Design review of the part built by this model. Coordinates are the model's own, in mm. A direction names the side the tool comes from. Give positions to 0.01 mm unless a question says otherwise; leave off trailing zeros. Write each loop counter-clockwise with the first axis right and the second up, starting at its lowest first coordinate (ties: lowest second). Pieces come first, ordered by that corner, then holes. Notation, with made-up numbers: (34, 19) -> (58, 19) arc R9 ccw to (58, 34) -> close; hole circle Ø1 at (62, 3.5). An arc over 180 degrees is marked (long way). Use CSV: the item, a comma, the result in double quotes.
```python
from build123d import *

# Parameters (mm, degrees)
F0_W     = 34
F0_H     = 16
F1_DEPTH = 58
F3_DEPTH = 38.001
F4_W     = 34
F4_H     = 11
F5_DEPTH = 16
F7_DEPTH = 10
F8_R     = 8
F9_DEPTH = 22


with BuildPart() as f1:
    # F0 (on Top) → F1 (new body)
    with BuildSketch(Plane.XY):
        Polygon((0, 38), (0, 0), (34, 0), (75, 0), (75, 38), align=None)
        with Locations((17, -8)):
            Rectangle(F0_W, F0_H)
        Polygon((85.358984, 38), (75, 38), (75, 0), (120, 0), (120, 18), align=None)
    extrude(amount=F1_DEPTH)

    # F2 (on face) → F3 (cut, through all)
    with BuildSketch(Plane.XZ):
        Polygon((75, 58), (120, 32.019238), (120, 58), align=None)
    extrude(amount=-F3_DEPTH, mode=Mode.SUBTRACT)

    # F4 (on face) → F5 (cut, symmetric)
    with BuildSketch(Plane.XZ.offset(16)):
        with Locations((17, 52.5)):
            Rectangle(F4_W, F4_H)
    extrude(amount=F5_DEPTH, both=True, mode=Mode.SUBTRACT)

    # F6 (on face) → F7 (join, symmetric)
    with BuildSketch(Plane.XZ.offset(16)):
        Polygon((34, 47), (0, 47), (0, 0), (5, 0), (5, -6), (29, -6), (29, 0), (34, 0), align=None)
    extrude(amount=F7_DEPTH, both=True)

    # F8 (on face) → F9 (cut)
    with BuildSketch(Plane.XZ.offset(26)):
        with Locations((17, 23.5)):
            Circle(F8_R)
    extrude(amount=-F9_DEPTH, mode=Mode.SUBTRACT)


solid = f1.part
```
(1) For line 1 along X through (y, z) = (-20, 23); line 2 along Z through (x, y) = (17, -9.5); line 3 along Y through (x, z) = (67.5, 39), list the stretches that pass through material, from the lowest coordinate up. Write a range as [from, to].
Established:
line 1,"x = [0, 9.02], [24.98, 34]"
line 2,"z = [-6, 15.5], [31.5, 47]"
line 3,"y = [0, 38]"
(2) Clearance check with flat-ended pins moving along their axes: pin 1 (3 mm diameter, centred on y = -18.5, z = -4, fed in from -X); pin 2 (1.8 mm diameter, centred on x = 19.5, z = -2, fed in from +Y); pin 3 (8 mm diameter, centred on x = 21.5, y = -17, fed in from +Z). State where each tip first meets the part, or that it passes through.
Established:
pin 1,"stops at x = 5"
pin 2,"stops at y = -6"
pin 3,"stops at z = 47"
(3) Take a section at C-C (x = 17). Write out the cut boundary in (y, z).
Established:
outline,"(-26, -6) -> (-6, -6) -> (-6, 0) -> (38, 0) -> (38, 58) -> (0, 58) -> (0, 47) -> (-26, 47) -> (-26, 31.5) -> (-4, 31.5) -> (-4, 15.5) -> (-26, 15.5) -> close"
(4) Tool access review of faces 1 (the face through (34, -13, 23)), 2 (the face through (5, -16, -3)), 3 (the face through (11.1, -15.2, 28.9)): name each direction out of +Z, -Z, +X, -X, +Y, -Y from which nothing blocks a thin tool from reaching the whole face with its end or side.
Established:
face 1,"+Z, -Z, +X, -Y"
face 2,"-Z, -X, +Y, -Y"
face 3,"-Y"
(5) Take a section at A-A (y = -10). Write out the cut boundary in (x, z), then the cut area to 3 significant figures.
Established:
outline,"(0, 0) -> (5, 0) -> (5, -6) -> (29, -6) -> (29, 0) -> (34, 0) -> (34, 47) -> (0, 47) -> close; hole circle Ø16 at (17, 23.5)"
area,"1,540 mm2"
(6) Take a section at D-D (y = 11). Write out the cut boundary in (x, z).
Established:
outline,"(0, 0) -> (120, 0) -> (120, 32.02) -> (75, 58) -> (0, 58) -> close"
(7) Take a section at B-B (z = 23.5). Write out the cut boundary in (x, y), then the cut area to 3 significant figures.
Established:
outline,"(0, -26) -> (9, -26) -> (9, -4) -> (25, -4) -> (25, -26) -> (34, -26) -> (34, 0) -> (120, 0) -> (120, 18) -> (85.36, 38) -> (0, 38) -> close"
area,"4,750 mm2"
(8) Mouldability with a two-part tool opening along Z and no side actions: class faces 4 (the face through (17, -13, 47)), 5 (the face through (17, -4, 24)), 6 (the face through (17, -26, 15)) as +Z half, -Z half, draft (parallel to the pull), parting line (faces both ways), or undercut.
Established:
face 4,"+Z half"
face 5,"undercut"
face 6,"draft"
